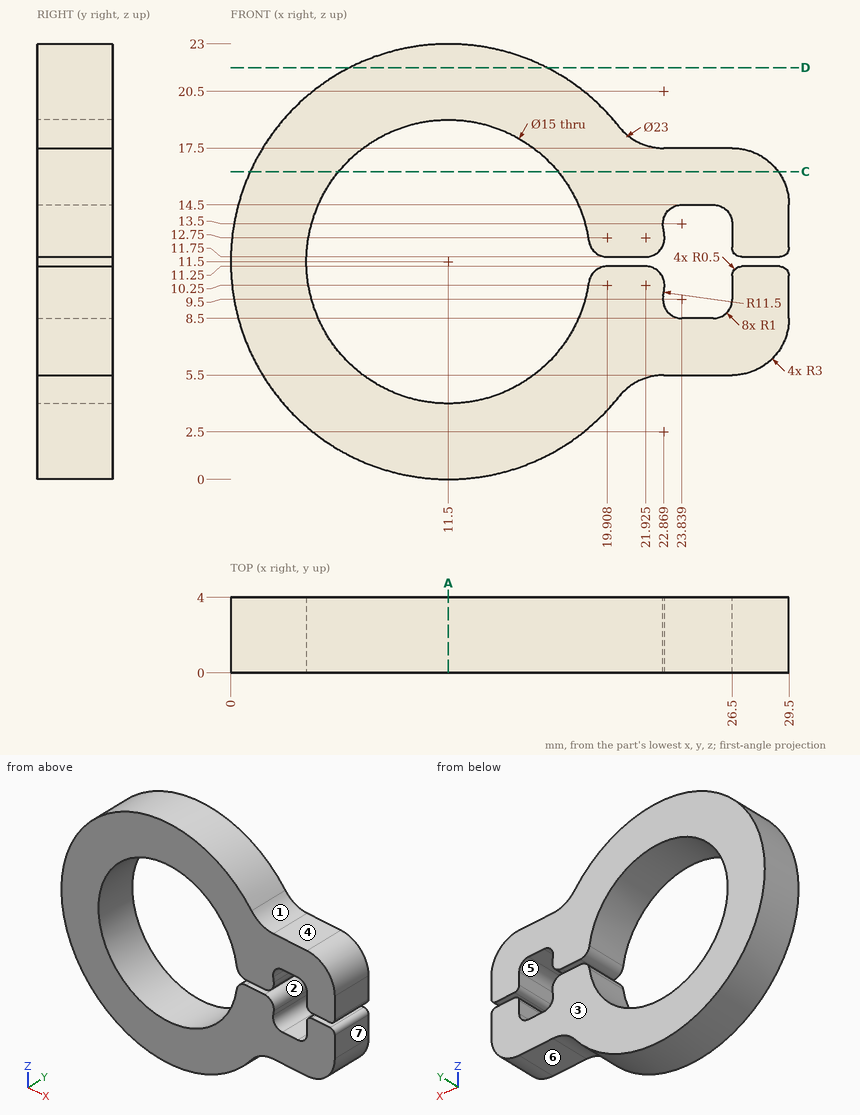
The drawing under review shows one solid part. Ordinate dimensions are in mm from its lowest x, y, z. A direction names the side the tool comes from. Give positions to 0.01 mm unless a question says otherwise; leave off trailing zeros. Write each loop counter-clockwise with the first axis right and the second up, starting at its lowest first coordinate (ties: lowest second). Pieces come first, ordered by that corner, then holes.
1. Draft analysis for pull direction X (two halves, no side actions). For the marked faces 1, 2 and 3, state which applies: +X half, -X half, draft (parallel to the pull), parting line (faces both ways), or undercut.
2. Wall thickness on L1, parallel to Z at x = 11.5, y = 3.05; L2, parallel to Z at x = 24.5, y = 0.6; L3, parallel to X at y = 3.5, z = 10.5: over which ranges is each line inside the solid? List them lowest first.
3. For P1, Ø9, axis at x = 11.5, z = 11.5, coming from the -Y side (3 decimals); P2, Ø1, axis at y = 1, z = 13, coming from the -X side; P3, Ø2, axis at y = 2.5, z = 16.5, coming from the -X side; P4, Ø2, axis at x = 28.5, y = 2.5, coming from the -Z side, all flat-tipped, find the tip position at first contact; note any pin that passes through.
4. Tool access review of the marked faces 4, 5, 6 and 7: name each direction out of +Z, -Z, +X, -X, +Y, -Y from which nothing blocks a thin tool from reaching the whole face with its end or side.
5. Add section C-C, the plane z = 16.25. Write out the cut boundary in (x, y).
6. Add section D-D, the plane z = 21.75. Write out the cut boundary in (x, y) (1 decimal).
7. Add section A-A, the plane x = 11.5. Write out the cut boundary in (y, z), plus the area to 3 significant figures.
Worked answers:
1. face 1: +X half
1. face 2: undercut
1. face 3: draft
2. L1: z = 0 to 4, 19 to 23
2. L2: z = 5.5 to 8.5, 14.5 to 17.5
2. L3: x = 0.04 to 4.07, 18.94 to 22.89, 26.5 to 29.5
3. P1: passes through
3. P2: stops at x = 0.04
3. P3: stops at x = 0.72
3. P4: stops at z = 5.67
4. face 4: +Z, +X, +Y, -Y
4. face 5: +Y, -Y
4. face 6: -Z, +X, +Y, -Y
4. face 7: +Z, -Z, +X, +Y, -Y
5. outline: (1.03, 0) - (5.7, 0) - (5.7, 4) - (1.03, 4) - close; (17.3, 0) - (28.94, 0) - (28.94, 4) - (17.3, 4) - close
6. outline: (6.3, 0) - (16.7, 0) - (16.7, 4) - (6.3, 4) - close
7. outline: (0, 0) - (4, 0) - (4, 4) - (0, 4) - close; (0, 19) - (4, 19) - (4, 23) - (0, 23) - close
7. area: 32.0 mm2
